Input: part model. Units: mm. Frame: model coordinates. Face numbers are marked on the shaded views. A direction names the side the tool comes from. Give positions to 0.01 mm unless a question says otherwise; leave off trailing zeros. Loops run counter-clockwise (first coordinate to the right, second up) from the corner with the lowest first, then second, coordinate; pieces in that order, holes last. Notation, with made-up numbers: M 65.5,51.25 L 123.5,51.25 A28 ccw 123.5,75.25 Z; hole C 68,26 d11. An arc over 180 degrees is marked long. Use CSV: the item, a comma, the result in double quotes. Start each with the question number.
Q1. Section D-D, the plane x = -21. Output: boundary loops of the cut face in (y, z) (3 decimals).
Q2. Material intervals for line 1 along Y through (x, z) = (-4, 9.5); line 2 along X through (y, z) = (17.5, 8.75) (3 decimals); line 3 along Z through (x, y) = (-1.5, 30), sorted ascending.
Q3. Section B-B, the plane x = 0. Output: boundary loops of the cut face in (y, z) (3 decimals).
Q4. Section C-C, the plane y = 6. Output: boundary loops of the cut face in (x, z) (3 decimals), plus the area to 3 significant figures.
Q5. Reachability of the marked faces 1, 2 and 3 from +Z, -Z, +X, -X, +Y, -Y: full face, straight path, thin tool, end or side. Return the list, or none.
Q6. Section A-A, the plane z = 0. Output: boundary loops of the cut face in (x, y) (3 decimals), plus the area to 3 significant figures.
Q7. Pin query (flat end, axial travel): pin 1 (12.5 mm diameter, centred on x = -6, z = 3.5, fed in from +Y); pin 2 (1 mm diameter, centred on x = -27.5, z = 1.5, fed in from +Y). Return the tip coordinate at first contact, or that it passes through.
from build123d import *

# Parameters (mm, degrees)
SKETCH_1_W          = 45.23
SKETCH_1_H          = 24.73
EXTRUDE_1_DEPTH     = 29
SKETCH_2_R          = 3
EXTRUDE_2_DEPTH     = 3.4
EXTRUDE_START       = 4.1
SKETCH_3_R          = 3
EXTRUDE_3_DEPTH     = 4.1
CUT_EXTRUDE_1_DEPTH = 50.815323446


with BuildPart() as part:
    # ｽｹｯﾁ1 → ﾎﾞｽ - 押し出し1 (new body)
    with BuildSketch(Plane(origin=(0, 0, 0), x_dir=(1, 0, 0), z_dir=(0, 1, 0))):
        with Locations((-12.5, 0)):
            Rectangle(SKETCH_1_W, SKETCH_1_H)
    extrude(amount=EXTRUDE_1_DEPTH)

    # ｽｹｯﾁ2 → ﾎﾞｽ - 押し出し2 (add)
    with BuildSketch(Plane(origin=(0, 29, 0), x_dir=(1, 0, 0), z_dir=(0, 1, 0))):
        with Locations(Location((0, 0, 0), (0, 0, 270))):
            Circle(SKETCH_2_R)
    extrude(amount=EXTRUDE_2_DEPTH)

    # ｽｹｯﾁ3 → ﾎﾞｽ - 押し出し3 (add)
    with BuildSketch(Plane.XZ.offset(EXTRUDE_START)):
        with Locations(Location((0, 0, 0), (0, 0, 90))):
            Circle(SKETCH_3_R)
    extrude(amount=-EXTRUDE_3_DEPTH)

    # ｽｹｯﾁ4 → ｶｯﾄ - 押し出し1 (cut, through all)
    with BuildSketch(Plane(origin=(0, 29, 0), x_dir=(1, 0, 0), z_dir=(0, 1, 0))):
        Polygon((5.31266953, 12.365), (10.115, 12.365), (10.115, 7.56266953), align=None)
        Polygon((5.31266953, -12.365), (10.115, -12.365), (10.115, -7.56266953), align=None)
    extrude(amount=-CUT_EXTRUDE_1_DEPTH, mode=Mode.SUBTRACT)


solid = part.part
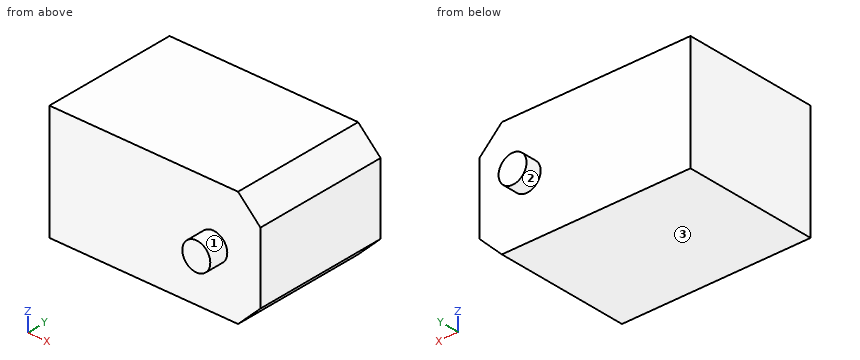
A:
1,outline,"M 0,-12.365 L 29,-12.365 L 29,12.365 L 0,12.365 Z"
2,line 1,"0 to 29"
2,line 2,"-35.115 to 8.928"
2,line 3,"-2.6 to 2.6"
3,outline,"M -4.1,-3 L 0,-3 L 0,-12.365 L 29,-12.365 L 29,-3 L 32.4,-3 L 32.4,3 L 29,3 L 29,12.365 L 0,12.365 L 0,3 L -4.1,3 Z"
4,outline,"M -35.115,-12.365 L 5.313,-12.365 L 10.115,-7.563 L 10.115,7.563 L 5.313,12.365 L -35.115,12.365 Z"
4,area,"1,100 mm^2"
5,face 1,"-Y"
5,face 2,"+Y"
5,face 3,"-Z, +X, -X, +Y, -Y"
6,outline,"M -35.115,0 L -3,0 L -3,-4.1 L 3,-4.1 L 3,0 L 10.115,0 L 10.115,29 L 3,29 L 3,32.4 L -3,32.4 L -3,29 L -35.115,29 Z"
6,area,"1,360 mm^2"
7,pin 1,"y = 32.4"
7,pin 2,"y = 29"
